from build123d import *

# Parameters (mm, degrees)
SKETCH1_R           = 1.5
BOSS_EXTRUDE1_DEPTH = 2
FILLET1_R           = 2
SKETCH2_R           = 1.5
SKETCH2_R_2         = 2.6
BOSS_EXTRUDE2_DEPTH = 2
CHAMFER1_SIZE       = 1
SKETCH3_R           = 1
BOSS_EXTRUDE3_DEPTH = 6
CHAMFER2_SIZE       = 3.5
CHAMFER2_SIZE2      = 0.4
SKETCH4_R           = 1.5
BOSS_EXTRUDE4_DEPTH = 2


with BuildPart() as part:
    # Sketch1 → Boss-Extrude1 (new body)
    with BuildSketch(Plane.XY):
        with BuildLine():
            Line((-2.75, -15), (-2.75, -6.15))
            Line((-2.75, -6.15), (-8.5, -6.15))
            Line((-8.5, -6.15), (-17.631690269, 1.463594463))
            ThreePointArc((-17.631690269, 1.463594463), (-18.665645679, 7.137466027), (-13.267909941, 9.168803324))
            Line((-13.267909941, 9.168803324), (-2.75, 5.5))
            Line((-2.75, 5.5), (6.5, 5.5))
            Line((6.5, 5.5), (6.5, -15))
            Line((6.5, -15), (-2.75, -15))
        make_face()
        Circle(SKETCH1_R, mode=Mode.SUBTRACT)
        with Locations((-14.75, 4.919872981)):
            Circle(SKETCH1_R, mode=Mode.SUBTRACT)
    extrude(amount=-BOSS_EXTRUDE1_DEPTH)

    # Fillet1
    fillet1_edges = [part.edges().sort_by_distance(p)[0] for p in [
        (6.5, -15, -1),
        (-2.75, -15, -1),
        (-2.75, -6.15, -1),
        (-8.5, -6.15, -1),
        (-2.75, 5.5, -1),
        (6.5, 5.5, -1),
    ]]
    fillet(fillet1_edges, radius=FILLET1_R)

    # Sketch2 → Boss-Extrude2 (add)
    with BuildSketch(Plane.XY):
        with BuildLine():
            Line((-0.75, -15), (4.5, -15))
            ThreePointArc((4.5, -15), (5.914213562, -14.414213562), (6.5, -13))
            Line((6.5, -13), (6.5, 3.5))
            ThreePointArc((6.5, 3.5), (5.914213562, 4.914213562), (4.5, 5.5))
            Line((4.5, 5.5), (-2.41119514, 5.5))
            ThreePointArc((-2.41119514, 5.5), (-2.745240817, 5.528093946), (-3.069901833, 5.611586514))
            Line((-3.069901833, 5.611586514), (-13.267909941, 9.168803324))
            ThreePointArc((-13.267909941, 9.168803324), (-18.665645679, 7.137466027), (-17.631690269, 1.463594463))
            Line((-17.631690269, 1.463594463), (-9.056369785, -5.686123786))
            ThreePointArc((-9.056369785, -5.686123786), (-8.456703141, -6.030458398), (-7.775618554, -6.15))
            Line((-7.775618554, -6.15), (-4.75, -6.15))
            ThreePointArc((-4.75, -6.15), (-3.335786438, -6.735786438), (-2.75, -8.15))
            Line((-2.75, -8.15), (-2.75, -13))
            ThreePointArc((-2.75, -13), (-2.164213562, -14.414213562), (-0.75, -15))
        make_face()
        Circle(SKETCH2_R, mode=Mode.SUBTRACT)
        with Locations((-14.75, 4.919872981)):
            Circle(SKETCH2_R_2, mode=Mode.SUBTRACT)
    extrude(amount=BOSS_EXTRUDE2_DEPTH)

    # Chamfer1
    chamfer1_edges = [part.edges().sort_by_distance(p)[0] for p in [
        (-2.164213562, -14.414213562, 2),
        (1.875, -15, 2),
        (5.914213562, -14.414213562, 2),
        (6.5, -4.75, 2),
        (5.914213562, 4.914213562, 2),
        (1.04440243, 5.5, 2),
        (-2.745240817, 5.528093946, 2),
        (-8.168905887, 7.390194919, 2),
        (-18.665645679, 7.137466027, 2),
        (-13.344030027, -2.111264661, 2),
        (-8.456703141, -6.030458398, 2),
        (-6.262809277, -6.15, 2),
        (-3.335786438, -6.735786438, 2),
        (-2.75, -10.575, 2),
    ]]
    chamfer(chamfer1_edges, length=CHAMFER1_SIZE)

    # Sketch3 → Boss-Extrude3 (add)
    with BuildSketch(Plane(origin=(0, 0, -2), x_dir=(-1, 0, 0), z_dir=(0, 0, -1))):
        with Locations(Location((0, -9.5, 0), (0, 0, 180))):
            Circle(SKETCH3_R)
    extrude(amount=BOSS_EXTRUDE3_DEPTH)

    # Chamfer2
    chamfer2_edges = [part.edges().sort_by_distance(p)[0] for p in [
        (-1, -9.5, -8),
    ]]
    chamfer2_side = [part.faces().sort_by_distance(p)[0] for p in [
        (-1, -9.5, -5),
    ]]
    chamfer(chamfer2_edges, length=CHAMFER2_SIZE, length2=CHAMFER2_SIZE2, reference=chamfer2_side[0])

    # Sketch4 → Boss-Extrude4 (add)
    with BuildSketch(Plane(origin=(0, 0, -2), x_dir=(-1, 0, 0), z_dir=(0, 0, -1))):
        with BuildLine():
            Line((13.267909941, 9.168803324), (8.168905887, 7.390194919))
            ThreePointArc((8.168905887, 7.390194919), (7.526785431, 6.683135075), (7.770894189, 5.759737426))
            Line((7.770894189, 5.759737426), (11.476857302, 1.831744604))
            ThreePointArc((11.476857302, 1.831744604), (19.121632111, 3.852711939), (13.267909941, 9.168803324))
        make_face()
        with Locations(Location((14.75, 4.919872981, 0), (0, 0, 180))):
            Circle(SKETCH4_R, mode=Mode.SUBTRACT)
    extrude(amount=BOSS_EXTRUDE4_DEPTH)


solid = part.part
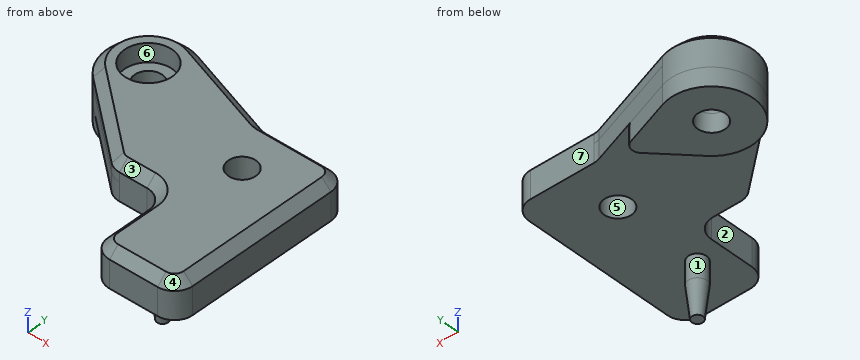
Source: CAD feature listing. Evaluate the final solid. Frame: model axes, mm. Face numbers are marked on the shaded views. A direction names the side the tool comes from. Round coordinates to 2 decimals unless told otherwise and drop trailing zeros. Loops run counter-clockwise (first coordinate to the right, second up) from the corner with the lowest first, then second, coordinate; pieces in that order, holes last. Notation, with made-up numbers: M -28.75,74 L -5.75,74 A20 ccw -5.75,113 Z; hole C 39.25,-18 d9. An arc over 180 degrees is marked long. Return JSON: item names as keys, results as strings. Group by question number.
1. Material intervals for line 1 along Y through (x, z) = (0, -0.3); line 2 along Y through (x, z) = (-14.75, -2.6); line 3 along Z through (x, y) = (-2, 4), sorted ascending. Write a range as from..to.
2. Pin query (flat end, axial travel): pin 1 (4 mm diameter, centred on x = 2, y = 5.5, fed in from -Z); pin 2 (4.5 mm diameter, centred on x = -11.5, y = 5, fed in from -Z); pin 3 (0.9 mm diameter, centred on x = 3, z = -0.5, fed in from +Y); pin 4 (1.8 mm diameter, centred on x = -14.75, y = 4.92, fed in from +Z). Return the tip coordinate at first contact, or that it passes through.
3. Reachability of the marked faces 1, 2 and 3 from +Z, -Z, +X, -X, +Y, -Y: full face, straight path, thin tool, end or side. Return the list, or none.
4. Section query C-C on z = 1.5. Output: boundary loops of the cut face in (x, y), and give its area (3 significant figures).
5. Section query B-B on y = 0. Output: boundary loops of the cut face in (x, z).
6. Section query D-D on y = -11.5. Output: boundary loops of the cut face in (x, z), and give its area (3 significant figures).
7. Section query A-A on x = 0. Output: boundary loops of the cut face in (y, z), and give its area (3 significant figures).
8. Mould query, pull axis Y, two halves, no side actions, for the marked faces 4, 5, 6 and 7. Classes: released by +Y, released by -Y, zero draft, split by the parting line, or undercut.
Checks:
{
 "1": {"line 1": "y = -15..-1.5, 1.5..5.5", "line 2": "y = 0.42..3.42, 6.42..9.42", "line 3": "z = -2..2"},
 "2": {"pin 1": "stops at z = -2", "pin 2": "stops at z = -4", "pin 3": "stops at y = 5.5", "pin 4": "passes through"},
 "3": {"face 1": "-Z", "face 2": "+Z, -Z, -X, -Y", "face 3": "+Z, -X, -Y"},
 "4": {"outline": "M -17.31,1.85 L -8.74,-5.3 A1.5 ccw -7.78,-5.65 L -4.75,-5.65 A2.5 cw -2.25,-8.15 L -2.25,-13 A1.5 ccw -0.75,-14.5 L 4.5,-14.5 A1.5 ccw 6,-13 L 6,3.5 A1.5 ccw 4.5,5 L -2.41,5 A2.5 cw -3.23,5.14 L -13.43,8.7 A4 ccw Z; hole C -14.75,4.92 d5.2; hole C 0,0 d3", "area": "299 mm²"},
 "5": {"outline": "M -15.88,-2 L -1.5,-2 L -1.5,2 L -14.31,2 L -15.88,1 Z; M 1.5,-2 L 6.5,-2 L 6.5,1 L 5.5,2 L 1.5,2 Z"},
 "6": {"outline": "M -2.75,-2 L 6.5,-2 L 6.5,1 L 5.5,2 L -1.75,2 L -2.75,1 Z", "area": "36.0 mm²"},
 "7": {"outline": "M -15,-2 L -10.5,-2 L -10.5,-4.5 L -10.1,-8 L -8.9,-8 L -8.5,-4.5 L -8.5,-2 L -1.5,-2 L -1.5,2 L -14,2 L -15,1 Z; M 1.5,-2 L 5.5,-2 L 5.5,1 L 4.5,2 L 1.5,2 Z", "area": "79.6 mm²"},
 "8": {"face 4": "released by -Y", "face 5": "undercut", "face 6": "undercut", "face 7": "released by +Y"}
}
